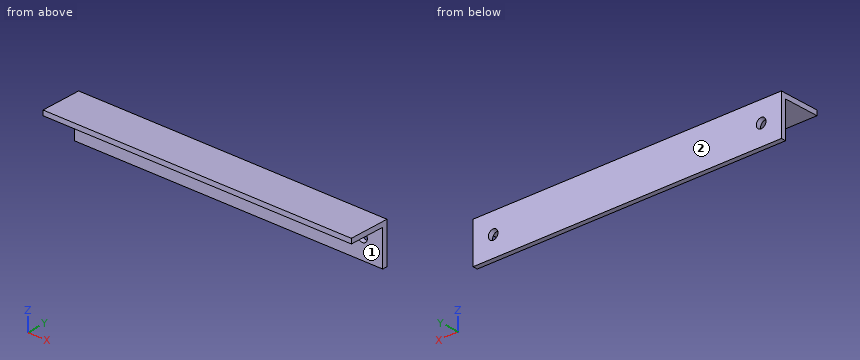
```python
from build123d import *

# Parameters (mm, degrees)
PAD_DEPTH               = 381.68773
COPYSKETCH001_R         = 6
POCKET_DEPTH            = 50.001
PADBODY_PITCH_ANGLE     = 90
PADBODY_PLACEMENT_ANGLE = -180


with BuildPart() as part:
    # Sketch → Pad (new body)
    with BuildSketch(Plane.XY):
        Polygon((0, 0), (0, 50), (6, 50), (6, 6), (50, 6), (50, 0), align=None)
    extrude(amount=PAD_DEPTH)

    # CopySketch001 (on Pad) → Pocket (cut, through all)
    with BuildSketch(Plane.XZ):
        with Locations((25, 25)):
            Circle(COPYSKETCH001_R)
        with Locations((25, 356.68773)):
            Circle(COPYSKETCH001_R)
    extrude(amount=-POCKET_DEPTH, mode=Mode.SUBTRACT)


with BuildPart() as part_1:
    # PadBody pitch: moved
    add(part.part.rotate(Axis((0, 0, 0), (0, 1, 0)), PADBODY_PITCH_ANGLE))


with BuildPart() as part_2:
    # PadBody placement: moved
    add(part_1.part.moved(Location((190.843865, 50, 0))).rotate(Axis((190.843865, 50, 0), (0, 0, 1)), PADBODY_PLACEMENT_ANGLE))


solid = part_2.part
```
Verification items for the finished model (mm, model axes). Face numbers are marked on the shaded views. A direction names the side the tool comes from. Coordinates: 2 decimals unless noted, no trailing zeros. Loops run counter-clockwise (first coordinate to the right, second up) from the corner with the lowest first, then second, coordinate; pieces in that order, holes last. Notation, with made-up numbers: (23.5, 53) -> (45.5, 53) arc R19 cw to (45.5, 76) -> close; hole circle Ø5 at (-39.5, 85.25). An arc over 180 degrees is marked (long way). Answer in a Markdown table with one row per item. Add a question column.
1. Section check B-B, the plane x = -118. Enter the section's corners in (y, z), then the cut area to 3 significant figures.
2. Section check C-C, the plane y = 4. Enter the section's corners in (x, z).
3. Access from +Z, -Z, +X, -X, +Y, -Y to the whole of each face (thin tool, end or side, straight path). Record for the marked faces 1 and 2.
4. Material ranges on probe 1 along X at (y, z) = (46, -25); probe 2 along Y at (x, z) = (89, -9.5); probe 3 along Z at (x, y) = (15.5, 13), recorded low to high. Write a range as [from, to].
5. Depth check by flat-ended pin: P1, Ø5, axis at x = -25, y = 5.5, coming from the -Z side; P2, Ø7, axis at x = 165.84, z = -25, coming from the -Y side; P3, Ø15.5, axis at x = -165.84, z = -25, coming from the -Y side. Enter the tip coordinate at first touch or a pass-through.
6. Section check A-A, the plane z = -25. Enter the section's corners in (x, y).
Derived:
| question | item | result |
|---|---|---|
| 1 | outline | (0, -6) -> (44, -6) -> (44, -50) -> (50, -50) -> (50, 0) -> (0, 0) -> close |
| 1 | area | 564 mm² |
| 2 | outline | (-190.84, -6) -> (190.84, -6) -> (190.84, 0) -> (-190.84, 0) -> close |
| 3 | face 1 | -Z, +X, -X, -Y |
| 3 | face 2 | +Z, -Z, +X, -X, +Y |
| 4 | probe 1 | x = [-190.84, -171.84], [-159.84, 159.84], [171.84, 190.84] |
| 4 | probe 2 | y = [44, 50] |
| 4 | probe 3 | z = [-6, 0] |
| 5 | P1 | stops at z = -6 |
| 5 | P2 | passes through |
| 5 | P3 | stops at y = 44 |
| 6 | outline | (-190.84, 44) -> (-171.84, 44) -> (-171.84, 50) -> (-190.84, 50) -> close; (-159.84, 44) -> (159.84, 44) -> (159.84, 50) -> (-159.84, 50) -> close; (171.84, 44) -> (190.84, 44) -> (190.84, 50) -> (171.84, 50) -> close |
